Could you check a few things on this model? Use its own coordinates, in mm. A direction names the side the tool comes from. Give positions to 0.01 mm unless a question says otherwise; leave off trailing zeros. Loops run counter-clockwise (first coordinate to the right, second up) from the corner with the lowest first, then second, coordinate; pieces in that order, holes last. Notation, with made-up numbers: M -16.75,56.5 L 5.25,56.5 A16 ccw 5.25,74.5 Z; hole C 34.5,22 d6. An arc over 180 degrees is marked long. Use a Markdown table: item, result. Add a question column.
1) Suppose I cut it at B-B on z = -9. List the corners of the cut face in (x, y) for me.
2) Which directions (+Z, -Z, +X, -X, +Y, -Y) give clear straight access to the entire face, cutting with the end or side of a thin tool? Please do faces 4 (the flat face through (-6, 16, 12)), 5 (the flat face through (-6, 20, -11)), 6 (the flat face through (-6, 20, 11)), 7 (the cylindrical face through (-7.587, 27.479, -6.186)), 8 (the flat face through (-6, 8, -11)).
3) Suppose I cut it at A-A on x = -0.75. List the corners of the cut face in (y, z) for me.
4) If I drill on line 1 along Z through (x, y) = (-0.75, 2.25); line 2 along Y through (x, z) = (-4.5, 12.5); line 3 along Y through (x, z) = (-10.75, 7), over which ranges is the centre line in solid material (lowest first)? Write a range as [from, to].
5) Will these pins go through, and if not, where does the flat tip stop? pin 1 Ø3 at (x, y) = (-8, 20.5) entering from +Z; pin 2 Ø3 at (y, z) = (24, 5) entering from -X; pin 3 Ø3 at (y, z) = (20, -1) entering from +X; pin 4 Ø4 at (x, z) = (-6, 14.18) entering from -Y.
6) Suppose I cut it at D-D on x = -2.5. List the corners of the cut face in (y, z) for me.
7) We'd pull the mould along X, two halves only. Please class faces 1 (the flat face through (-3, 17, -16)), 2 (the cylindrical face through (-6.05, 23.97, -10.97)), 3 (the cylindrical face through (-5.941, 17.014, 12.685)): +X half, -X half, draft (parallel to the pull), parting line (faces both ways), or undercut.
8) Suppose I cut it at C-C on y = 8. List the corners of the cut face in (x, z) for me.
Autodesk Inventor part; units mm, degrees
ref_plane "YZ Plane" through (0, 0, 0) normal (1, 0, 0) x (0, 1, 0)
ref_plane "XZ Plane" through (0, 0, 0) normal (0, 1, 0) x (-1, 0, 0)
ref_plane "XY Plane" through (0, 0, 0) normal (0, 0, 1) x (1, 0, 0)
sketch "Boceto1" plane through (0, 0, 0) normal (0, 1, 0) x (-1, 0, 0)
  line L0 (0, 0) -> (12, 0)
  line L1 (12, 0) -> (12, -11)
  line L2 (12, -11) -> (0, -11)
  line L3 (0, -11) -> (0, 0)
extrude "Extrusión1" add sketch "Boceto1" along normal blind 22
sketch "Boceto2" plane through (0, 0, -11) normal (0, 0, -1) x (-1, 0, 0)
  line L0 (12, 22) -> (0, 22)
  line L1 (0, 18) -> (12, 18)
  line L2 (0, 16) -> (12, 16)
  line L3 (12, 0) -> (12, 22)
  line L4 (0, 18) -> (0, 16)
  line L5 (0, 0) -> (0, 22)
  line L6 (12, 18) -> (12, 16)
extrude "Extrusión2" add sketch "Boceto2" along normal blind 5 contours L3 L2 L4 L1
sketch "Boceto3" plane through (-12, 18, -11) normal (0, 1, 0) x (1, 0, 0)
  line L0 (0, 5) -> (12, 5)
  arc A0 (5.5, 4.5976) -> (6.5, 4.5976) centre (6, 3.1834) ccw
  line L1 (5.5, 4.5976) -> (5.5, 5)
  line L2 (5.5, 5) -> (6.5, 5)
  line L3 (6.5, 4.5976) -> (6.5, 5)
  point P0 (12, -11)
extrude "Extrusión3" cut sketch "Boceto3" against normal through all
mirror "Simetría1" about plane through (-12, 0, 0) normal (0, 0, 1) of "Extrusión1", "Extrusión2", "Extrusión3"
sketch "Boceto5" plane through (0, 22, 0) normal (0, 1, 0) x (1, 0, 0)
  line L0 (0, 11) -> (-12, 11)
  arc A0 (-3.6616, -0.5562) -> (-8.6574, -0.41) centre (-6, 4.9694) ccw
  arc A1 (-8.6574, -0.41) -> (-3.6616, -0.5562) centre (-6.1574, -0.412) ccw
  point P0 (0, 0)
extrude "Extrusión4" add sketch "Boceto5" along normal blind 4
sketch "Boceto6" plane through (0, 26, 0) normal (0, 1, 0) x (1, 0, 0)
  line L0 (0, 11) -> (0, 4.9694)
  arc A0 (0, 4.9694) -> (-12, 4.9694) centre (-6, 4.9694) ccw
  circle A1 centre (-6, 4.9694) radius 2
  point P0 (0, 0)
extrude "Extrusión5" add sketch "Boceto6" along normal blind 3
equation "\"Radio_pliegue\" = Grosor"
equation "\"Anchura_desahogo_plegado\" = Grosor"
equation "\"Profundidad_desahogo_plegado\" = 0.5 * Grosor"
equation "\"Tamaño_destalonado\" = 4 * Grosor"
equation "\"Remanente_mínimo\" = 2 * Grosor"
equation "\"Radiodetransición\" = Radio_pliegue"
equation "\"Tamaño_de_radio_de_Jacobi\" = Radio_pliegue"
equation "\"TamañoSeparación\" = Grosor"
properties part number "servo"
Answer block:
| question | item | result |
|---|---|---|
| 1 | outline | M -12,0 L 0,0 L 0,22 L -1.56,22 L -1.56,26 L -10.44,26 L -10.44,22 L -12,22 Z |
| 2 | face 4 | +Z, +X, -X, -Y |
| 2 | face 5 | -Z, +X, -X, +Y |
| 2 | face 6 | +Z, +X, -X, +Y |
| 2 | face 7 | +Y |
| 2 | face 8 | -Z, +X, -X, -Y |
| 3 | outline | M 0,-11 L 16,-11 L 16,-16 L 18,-16 L 18,-11 L 22,-11 L 22,-7.87 L 26,-7.87 L 26,-2.06 L 22,-2.06 L 22,11 L 18,11 L 18,16 L 16,16 L 16,11 L 0,11 Z |
| 4 | line 1 | z = [-11, 11] |
| 4 | line 2 | y = [16, 18] |
| 4 | line 3 | y = [0, 22] |
| 5 | pin 1 | stops at z = 11 |
| 5 | pin 2 | passes through |
| 5 | pin 3 | stops at x = 0 |
| 5 | pin 4 | stops at y = 16 |
| 6 | outline | M 0,-11 L 16,-11 L 16,-16 L 18,-16 L 18,-11 L 22,-11 L 22,-9.84 L 26,-9.84 L 26,-0.1 L 22,-0.1 L 22,11 L 18,11 L 18,16 L 16,16 L 16,11 L 0,11 Z |
| 7 | face 1 | draft |
| 7 | face 2 | parting line |
| 7 | face 3 | undercut |
| 8 | outline | M -12,-11 L 0,-11 L 0,11 L -12,11 Z |
